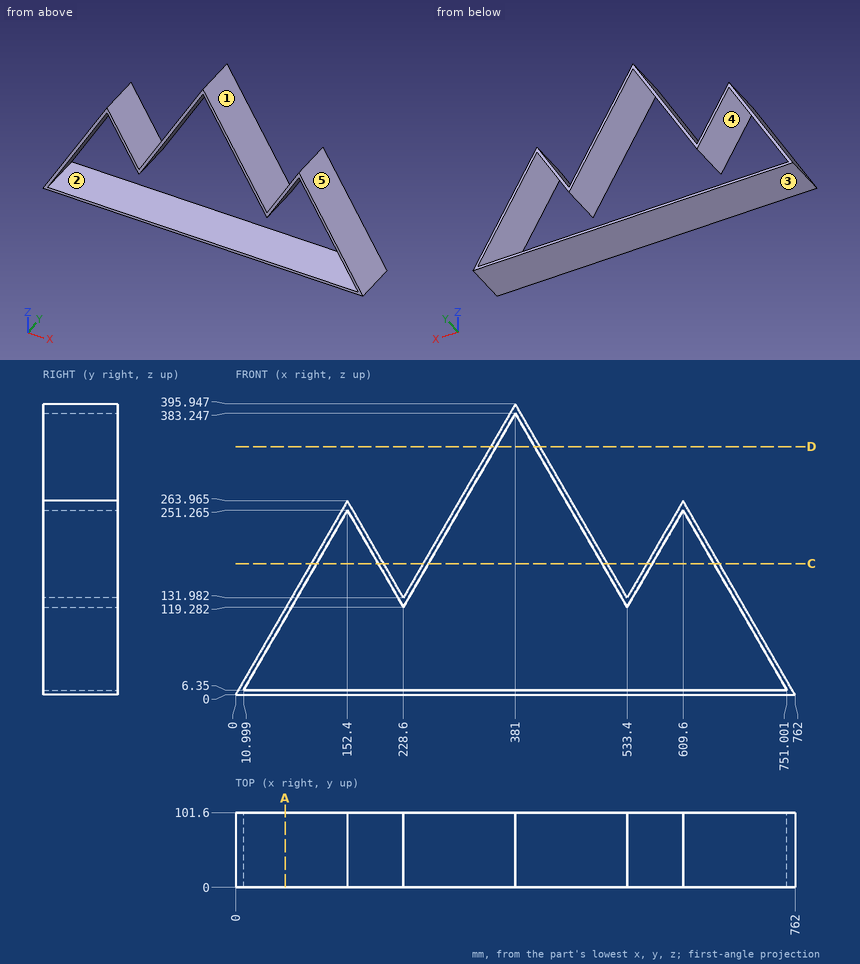
Could you check a few things on this drawing? It's one solid part, dimensions in mm from its lowest x, y, z. A direction names the side the tool comes from. Round coordinates to 2 decimals unless told otherwise and drop trailing zeros. Order: outer loops, then holes, each group sorted by start corner. A loop starts at its lowest first (then second) coordinate and runs counter-clockwise, first axis right, second up. Notation, with made-up numbers: M 79,27 L 101,27 A21 ccw 101,58 Z; hole C -13,31.5 d1. An arc over 180 degrees is marked long. Use a Markdown table: item, result.
1) I'm going to push flat-ended pins straight in: P1, Ø8, axis at y = 14.5, z = 44, coming from the +X side (1 decimal); P2, Ø5, axis at y = 91.5, z = 234.5, coming from the +X side (1 decimal); P3, Ø4, axis at x = 630.5, y = 64.5, coming from the +Z side; P4, Ø10, axis at x = 443.5, z = 295.5, coming from the -Y side. Where does each tip first touch, or does it pass through?
Geometry says:
| item | result |
|---|---|
| P1 | stops at x = 738.9 |
| P2 | stops at x = 628.1 |
| P3 | stops at z = 231.23 |
| P4 | stops at y = 0 |
2) Imagine slicing it at C-C (z = 178.5). List the corners of the cut face in (x, y) for me, then the cut area to 3 significant figures.
Geometry says:
| item | result |
|---|---|
| outline | M 103.06,0 L 110.39,0 L 110.39,101.6 L 103.06,101.6 Z; M 194.41,0 L 201.74,0 L 201.74,101.6 L 194.41,101.6 Z; M 255.46,0 L 262.79,0 L 262.79,101.6 L 255.46,101.6 Z; M 499.21,0 L 506.54,0 L 506.54,101.6 L 499.21,101.6 Z; M 560.26,0 L 567.59,0 L 567.59,101.6 L 560.26,101.6 Z; M 651.61,0 L 658.94,0 L 658.94,101.6 L 651.61,101.6 Z |
| area | 4,470 mm² |
3) If we mould it in two halves opening along X, with no side actions, what happens to the marked faces 3, 4 and 5? For each: +X half, -X half, draft (parallel to the pull), parting line (faces both ways), or undercut.
Geometry says:
| item | result |
|---|---|
| face 3 | draft |
| face 4 | undercut |
| face 5 | +X half |
4) If I drill on line 1 along X through (y, z) = (42, 263) (1 decimal); line 2 along X through (y, z) = (97.5, 230.5); line 3 along X through (y, z) = (96.5, 259) (1 decimal), over which ranges is the centre line in solid material (lowest first)?
Geometry says:
| item | result |
|---|---|
| line 1 | x = 151.8 to 153, 304.2 to 311.6, 450.4 to 457.8, 609 to 610.2 |
| line 2 | x = 133.08 to 140.41, 164.39 to 171.72, 285.48 to 292.81, 469.19 to 476.52, 590.28 to 597.61, 621.59 to 628.92 |
| line 3 | x = 149.5 to 155.3, 301.9 to 309.3, 452.7 to 460.1, 606.7 to 612.5 |
5) Imagine slicing it at A-A (x = 67.5). List the corners of the cut face in (y, z) for me, then the cut area to 3 significant figures.
Geometry says:
| item | result |
|---|---|
| outline | M 0,0 L 101.6,0 L 101.6,6.35 L 0,6.35 Z; M 0,104.21 L 101.6,104.21 L 101.6,116.91 L 0,116.91 Z |
| area | 1,940 mm² |
6) On a 3-axis mill with a long thin cutter (end or side, diameter ignored), from which of +Z, -Z, +X, -X, +Y, -Y can I reach the whole of each face in a straight line? I mean the marked faces 1 and 2. Say none if no direction works.
Geometry says:
| item | result |
|---|---|
| face 1 | +Z, +Y, -Y |
| face 2 | +Y, -Y |
7) Imagine slicing it at D-D (z = 338). List the corners of the cut face in (x, y) for me (1 decimal), then the cut area to 3 significant figures.
Geometry says:
| item | result |
|---|---|
| outline | M 347.5,0 L 354.9,0 L 354.9,101.6 L 347.5,101.6 Z; M 407.1,0 L 414.5,0 L 414.5,101.6 L 407.1,101.6 Z |
| area | 1,490 mm² |
